Autodesk Inventor part; units mm, degrees
ref_plane "YZ Plane" through (0, 0, 0) normal (1, 0, 0) x (0, 1, 0)
ref_plane "XZ Plane" through (0, 0, 0) normal (0, 1, 0) x (-1, 0, 0)
ref_plane "XY Plane" through (0, 0, 0) normal (0, 0, 1) x (1, 0, 0)
sketch "Sketch1" plane through (0, 0, 0) normal (0, 0, 1) x (1, 0, 0)
  line L0 (0, 0) -> (14, 0)
  line L1 (14, 0) -> (14, -14)
  line L2 (14, -14) -> (0, -14)
  line L3 (0, -14) -> (0, 0)
  dimension "d0" = 14
  dimension "d1" = 14
extrude "Extrusion1" add sketch "Sketch1" against normal blind 22
sketch "Sketch2" plane through (0, 0, 0) normal (0, 0, 1) x (1, 0, 0)
  line L0 (2, -2) -> (12, -2)
  line L1 (12, -2) -> (12, -22)
  line L2 (12, -22) -> (2, -22)
  line L3 (2, -22) -> (2, -2)
  point P0 (0, 0)
  dimension "d4" = 10
  dimension "d5" = 20
extrude "Extrusion2" cut sketch "Sketch2" against normal blind 20
sketch "Sketch8" plane through (0, -14, 0) normal (-1, 0, 0) x (0, 0, 1)
  point P0 (0, 14)
sketch "Sketch9" plane through (0, -14, 0) normal (-1, 0, 0) x (0, 0, 1)
  point P0 (0, 14)
sketch "Sketch11" plane through (0, -14, 0) normal (-1, 0, 0) x (0, 0, 1)
  point P0 (0, 14)
sketch "Sketch14" plane through (0, -14, 0) normal (-1, 0, 0) x (0, 0, 1)
  point P0 (0, 14)
sketch "Sketch15" plane through (0, -14, 0) normal (-1, 0, 0) x (0, 0, 1)
  point P0 (0, 14)
sketch "Sketch16" plane through (0, -14, 0) normal (-1, 0, 0) x (0, 0, 1)
  line L0 (-12.5, 12) -> (-17.5, 12)
  line L1 (-17.5, 12) -> (-17.5, 0)
  line L2 (-17.5, 0) -> (-12.5, 0)
  line L3 (-12.5, 0) -> (-12.5, 12)
  point P0 (0, 14)
  dimension "d30" = 5
  dimension "d31" = 12
extrude "Extrusion10" cut sketch "Sketch16" against normal blind 2
sketch "Sketch17" plane through (0, 0, -20) normal (0, 0, 1) x (1, 0, 0)
  line L0 (12, -2) -> (7.5, -2)
  line L1 (7.5, -2) -> (7.5, -5.5)
  line L2 (7.5, -5.5) -> (12, -5.5)
  line L3 (12, -5.5) -> (12, -2)
  point P0 (0, 0)
  dimension "d34" = 4.5
  dimension "d35" = 3.5
extrude "Extrusion11" add sketch "Sketch17" along normal blind 9
fillet "Fillet1" radius 0.8 8 edges at (0, -8, -12.5) (2, -8, -12.5) (0, -2, -15) (0, -8, -17.5) (2, -8, -17.5) (12, -14, -10) (7.5, -5.5, -15.5) (9.75, -5.5, -11)
properties part number "housing_v09"
Design review of the part built by this model. Coordinates are the model's own, in mm. A direction names the side the tool comes from. Round coordinates to 2 decimals unless told otherwise and drop trailing zeros. Loops run counter-clockwise (first coordinate to the right, second up) from the corner with the lowest first, then second, coordinate; pieces in that order, holes last. Notation, with made-up numbers: (16.5, 41.25) -> (62.5, 41.25) arc R17 ccw to (62.5, 74.25) -> close; hole circle Ø11 at (60.5, 51.5). An arc over 180 degrees is marked (long way). Use one line per item in the form item = value. Start each with the question number.
Q1. We need section A-A on y = -4. Give the boundary of the cut face in (x, z), then the cut area to 3 significant figures.
Q2. Draft analysis for pull direction Z (two halves, no side actions). For faces 5 (the face through (7, -7, -22)), 6 (the face through (6, -8, -20)), 7 (the face through (1, -14, -6)), 8 (the face through (0.24, -7.69, -17.73)), state which applies: +Z half, -Z half, draft (parallel to the pull), parting line (faces both ways), or undercut.
Q3. Machinability: for faces 1 (the face through (0.24, -7.51, -12.27)), 2 (the face through (10, -5.5, -16)), 3 (the face through (1.77, -8.08, -17.74)), 4 (the face through (0, -7, -8)), which of the approach directions +Z, -Z, +X, -X, +Y, -Y give a long, thin tool a straight path to every point of the face, cutting with its end or side? Answer none if there is none.
Q4. We need section D-D on y = -11. Give the boundary of the cut face in (x, z), then the cut area to 3 significant figures.
Q5. We need section C-C on z = -4. Give the boundary of the cut face in (x, y), then the cut area to 3 significant figures.
Q6. For pin 1 Ø1 at (x, z) = (3, -8.5) entering from -Y; pin 2 Ø1.1 at (x, z) = (10, -17.5) entering from -Y; pin 3 Ø0.8 at (y, z) = (-3, -16.5) entering from -X, all flat-tipped, find the tip position at first contact; note any pin that passes through.
Q7. Wall thickness on line 1 along X through (y, z) = (-10, -9.75); line 2 along Z through (x, y) = (1, -12.5); line 3 along Y through (x, z) = (11.5, -13): over which ranges is each line inside the solid? List them lowest first. Write a range as [from, to].
Q8. We need section B-B on x = 11.5. Give the boundary of the cut face in (y, z), then the cut area to 3 significant figures.
Calculated:
q1.outline = (0, -22) -> (14, -22) -> (14, 0) -> (12, 0) -> (12, -11) -> (7.5, -11) -> (7.5, -20) -> (2, -20) -> (2, -18.3) arc R0.8 ccw to (1.2, -17.5) -> (0.8, -17.5) arc R0.8 ccw to (0, -18.3) -> close; (0, -11.7) arc R0.8 ccw to (0.8, -12.5) -> (1.2, -12.5) arc R0.8 ccw to (2, -11.7) -> (2, 0) -> (0, 0) -> close
q1.area = 138 mm²
q2.face_5 = -Z half
q2.face_6 = +Z half
q2.face_7 = draft
q2.face_8 = undercut
q3.face_1 = -X, -Y
q3.face_2 = +Z, -Y
q3.face_3 = -Y
q3.face_4 = +Z, -Z, -X, +Y, -Y
q4.outline = (0, -22) -> (14, -22) -> (14, 0) -> (12, 0) -> (12, -20) -> (2, -20) -> (2, -18.3) arc R0.8 ccw to (1.2, -17.5) -> (0.8, -17.5) arc R0.8 ccw to (0, -18.3) -> close; (0, -11.7) arc R0.8 ccw to (0.8, -12.5) -> (1.2, -12.5) arc R0.8 ccw to (2, -11.7) -> (2, 0) -> (0, 0) -> close
q4.area = 97.5 mm²
q5.outline = (0, -14) -> (2, -14) -> (2, -2) -> (12, -2) -> (12, -13.2) arc R0.8 ccw to (12.8, -14) -> (14, -14) -> (14, 0) -> (0, 0) -> close
q5.area = 75.9 mm²
q6.pin_1 = -2
q6.pin_2 = -5.5
q6.pin_3 = 7.5
q7.line_1 = [0, 2], [12, 14]
q7.line_2 = [-22, -17.5], [-12.5, 0]
q7.line_3 = [-5.5, 0]
q8.outline = (-14, -22) -> (0, -22) -> (0, 0) -> (-2, 0) -> (-2, -11) -> (-4.7, -11) arc R0.8 ccw to (-5.5, -11.8) -> (-5.5, -20) -> (-14, -20) -> close
q8.area = 99.4 mm²
